```python
from build123d import *

# Parameters (mm, degrees)
SKETCH1_W                                      = 350
SKETCH1_H                                      = 350
SKETCH1_R                                      = 3.2
BASE_PLATE_STRUCTURAL_PANEL_DEPTH              = 1.5
SKETCH2_W                                      = 310
SKETCH2_H                                      = 310
SKETCH2_W_2                                    = 302.8
SKETCH2_H_2                                    = 302.8
BASE_PLATE_STRUCTURAL_PANEL_INSET_STIFFE_DEPTH = 1.9


with BuildPart() as part:
    # Sketch1 → Base plate structural panel (new, symmetric)
    with BuildSketch(Plane(origin=(0, 0, 0), x_dir=(1, 0, 0), z_dir=(0, 1, 0))):
        Rectangle(SKETCH1_W, SKETCH1_H)
        with Locations(Location((164, 164, 0), (0, 0, 270))):
            Circle(SKETCH1_R, mode=Mode.SUBTRACT)
        with Locations(Location((-164, 164, 0), (0, 0, 270))):
            Circle(SKETCH1_R, mode=Mode.SUBTRACT)
        with Locations(Location((164, -164, 0), (0, 0, 270))):
            Circle(SKETCH1_R, mode=Mode.SUBTRACT)
        with Locations(Location((-164, -164, 0), (0, 0, 270))):
            Circle(SKETCH1_R, mode=Mode.SUBTRACT)
    extrude(amount=BASE_PLATE_STRUCTURAL_PANEL_DEPTH, both=True)

    # Sketch2 → Base plate structural panel inset stiffener (add, symmetric)
    with BuildSketch(Plane(origin=(0, 0, 0), x_dir=(1, 0, 0), z_dir=(0, 1, 0))):
        Rectangle(SKETCH2_W, SKETCH2_H)
        Rectangle(SKETCH2_W_2, SKETCH2_H_2, mode=Mode.SUBTRACT)
    extrude(amount=BASE_PLATE_STRUCTURAL_PANEL_INSET_STIFFE_DEPTH, both=True)


solid = part.part
```
Could you check a few things on this model? Use its own coordinates, in mm. Round coordinates to 2 decimals unless told otherwise and drop trailing zeros. Loops run counter-clockwise (first coordinate to the right, second up) from the corner with the lowest first, then second, coordinate; pieces in that order, holes last. Notation, with made-up numbers: (41.5, 39) -> (63.5, 39) arc R21 cw to (63.5, 59) -> close; hole circle Ø4 at (68, 76). An arc over 180 degrees is marked (long way). One line per question, with ' | ' between items.
(1) For pin 1 Ø6 at (x, z) = (30.5, -94) entering from +Y; pin 2 Ø1 at (x, z) = (109, 15) entering from -Y; pin 3 Ø4 at (x, z) = (164, 164) entering from +Y, each with a flat end and sliding along its axis, tell me the tip position at first contact or that it passes through.
Model answer:
pin 1: stops at y = 1.5 | pin 2: stops at y = -1.5 | pin 3: passes through
(2) Thinking about a two-plate mould opening in Z: for faces 1 (the face through (-2, -1.5, -2)), 2 (the face through (-2, 1.5, -2)), 3 (the face through (-156, -1.5, -27)), which applies, released by +Z, released by -Z, zero draft, split by the parting line, or undercut?
Model answer:
face 1: undercut | face 2: undercut | face 3: zero draft
(3) If I drill on probe 1 along Z at (x, y) = (164, 0.15); probe 2 along X at (y, z) = (1.6, -129.5), over which ranges is the centre line in solid material (lowest first)?
Model answer:
probe 1: z = -175 to -167.2, -160.8 to 160.8, 167.2 to 175 | probe 2: x = -155 to -151.4, 151.4 to 155
(4) If we section it at B-B on x = -60: List the corners of the cut face in (y, z) for me.
Model answer:
outline: (-1.9, -155) -> (-1.5, -155) -> (-1.5, -175) -> (1.5, -175) -> (1.5, -155) -> (1.9, -155) -> (1.9, -151.4) -> (1.5, -151.4) -> (1.5, 151.4) -> (1.9, 151.4) -> (1.9, 155) -> (1.5, 155) -> (1.5, 175) -> (-1.5, 175) -> (-1.5, 155) -> (-1.9, 155) -> (-1.9, 151.4) -> (-1.5, 151.4) -> (-1.5, -151.4) -> (-1.9, -151.4) -> close
(5) If we section it at A-A on z = 84.5: List the corners of the cut face in (x, y) for me.
Model answer:
outline: (-175, -1.5) -> (-155, -1.5) -> (-155, -1.9) -> (-151.4, -1.9) -> (-151.4, -1.5) -> (151.4, -1.5) -> (151.4, -1.9) -> (155, -1.9) -> (155, -1.5) -> (175, -1.5) -> (175, 1.5) -> (155, 1.5) -> (155, 1.9) -> (151.4, 1.9) -> (151.4, 1.5) -> (-151.4, 1.5) -> (-151.4, 1.9) -> (-155, 1.9) -> (-155, 1.5) -> (-175, 1.5) -> close
